Here's how the part is built. I have some questions about the finished solid (model axes, mm). A direction names the side the tool comes from. Give positions to 0.01 mm unless a question says otherwise; leave off trailing zeros. Write each loop counter-clockwise with the first axis right and the second up, starting at its lowest first coordinate (ties: lowest second). Pieces come first, ordered by that corner, then holes. Notation, with made-up numbers: (-36, -36.5) - (10, -36.5) arc R21 ccw to (10, -17.5) - close; hole circle Ø8 at (50.25, 22.25). An arc over 180 degrees is marked (long way). Write each question's results on one line, items separated by ' | '. Start each with the question number.
Item 1: Which directions (+Z, -Z, +X, -X, +Y, -Y) give clear straight access to the entire face, cutting with the end or side of a thin tool? Please do faces 1 (the flat face through (-102.855, 11, 2)), 2 (the flat face through (-101, -5.5, 2)), 3 (the flat face through (-24, -20.5, 3)).
Item 2: Suppose I cut it at C-C on x = -72.5. List the corners of the cut face in (y, z) for me, then the cut area to 3 significant figures.
Item 3: Suppose I cut it at A-A on z = 7.5. List the corners of the cut face in (x, y) for me.
Item 4: Will these pins go through, and if not, where does the flat tip stop? P1, Ø4, axis at x = -54.5, y = -14.5, coming from the +Z side; P2, Ø0.6, axis at x = -100.5, z = 10, coming from the +Y side; P3, Ø2.5, axis at x = 49, z = 8.5, coming from the -Y side.
Item 5: Suppose I cut it at B-B on y = -17.5. List the corners of the cut face in (x, z) for me.
Item 6: Please list where these lines run through material, in increasing order: line 1 along Y through (x, z) = (-8.5, 3); line 2 along X through (y, z) = (-16, 2.75); line 3 along X through (y, z) = (-8, 3.5).
Item 7: Suppose I cut it at D-D on y = 8. List the corners of the cut face in (x, z) for me.
Item 8: We'd pull the mould along Y, two halves only. Please class faces 4 (the flat face through (-102.855, -14, 2)), 5 (the flat face through (-26, -23.5, 2)), 6 (the flat face through (-26, -10.5, 3)): +Y half, -Y half, draft (parallel to the pull), parting line (faces both ways), or undercut.
```python
from build123d import *

# Parameters (mm, degrees)
F0_W     = 150
F0_H     = 3
F1_DEPTH = 5
F0_H_2   = 7
F2_DEPTH = 2
F3_DEPTH = 11
F5_W     = 2
F5_H     = 2
F6_DEPTH = 2
F7_R     = 1.5
F8_W     = 2
F8_H     = 2
F9_DEPTH = 2
F10_R    = 1.8


with BuildPart() as f1:
    # F0 (on Top) → F1 (new body)
    with BuildSketch(Plane.XY):
        Polygon((53.1447380781, 19.5), (-102.8552619219, 19.5), (-102.8552619219, 1.5), (-99.8552619219, 1.5), (-99.8552619219, 4.5), (-99.8552619219, 6.5), (-99.8552619219, 9.5), (-99.8552619219, 16.5), (50.1447380781, 16.5), (50.1447380781, 9.5), (50.1447380781, 6.5), (50.1447380781, 3), (50.1447380781, 0), (53.1447380781, 0), align=None)
        Polygon((-99.8552619219, 4.5), (-99.8552619219, 1.5), (-99.8552619219, -5.5), (-99.8552619219, -8.5), (-96.8552619219, -8.5), (-96.8552619219, 4.5), align=None)
        Polygon((-99.8552619219, -5.5), (-102.8552619219, -5.5), (-102.8552619219, -23.5), (53.1447380781, -23.5), (53.1447380781, -4), (50.1447380781, -4), (50.1447380781, -7), (50.1447380781, -10.5), (50.1447380781, -13.5), (50.1447380781, -20.5), (-99.8552619219, -20.5), (-99.8552619219, -13.5), (-99.8552619219, -10.5), (-99.8552619219, -8.5), align=None)
        with Locations((-24.8552619219, -12)):
            Rectangle(F0_W, F0_H)
        with Locations((-24.8552619219, 8)):
            Rectangle(F0_W, F0_H)
        Polygon((50.1447380781, -4), (50.1447380781, 0), (50.1447380781, 3), (47.1447380781, 3), (47.1447380781, -7), (50.1447380781, -7), align=None)
    extrude(amount=F1_DEPTH)

    # F0 (on Top) → F2 (join)
    with BuildSketch(Plane.XY):
        with Locations((-24.8552619219, 13)):
            Rectangle(F0_W, F0_H_2)
        Polygon((-99.8552619219, 6.5), (-99.8552619219, 4.5), (-96.8552619219, 4.5), (-96.8552619219, -8.5), (-99.8552619219, -8.5), (-99.8552619219, -10.5), (50.1447380781, -10.5), (50.1447380781, -7), (47.1447380781, -7), (47.1447380781, 3), (50.1447380781, 3), (50.1447380781, 6.5), align=None)
        with Locations((-24.8552619219, -17)):
            Rectangle(F0_W, F0_H_2)
    extrude(amount=F2_DEPTH)


with BuildPart() as f3:
    # F0 (on Top) → F3 (new body)
    with BuildSketch(Plane.XY):
        Polygon((-99.8552619219, 4.5), (-99.8552619219, 1.5), (-99.8552619219, -5.5), (-99.8552619219, -8.5), (-96.8552619219, -8.5), (-96.8552619219, 4.5), align=None)
    extrude(amount=F3_DEPTH)


with BuildPart() as f3b:
    # F0 (on Top) → F3, piece 2 (new body)
    with BuildSketch(Plane.XY):
        Polygon((50.1447380781, -4), (50.1447380781, 0), (50.1447380781, 3), (47.1447380781, 3), (47.1447380781, -7), (50.1447380781, -7), align=None)
    extrude(amount=F3_DEPTH)


with BuildPart() as f1_1:
    add(f1.part)

    # F4: union F3b, F3
    add(f3b.part)
    add(f3.part)

    # F5 (on face) → F6 (join)
    with BuildSketch(Plane(origin=(-99.8552619219, 0, 0), x_dir=(0, -1, 0), z_dir=(-1, 0, 0))):
        with Locations((2, 10)):
            Rectangle(F5_W, F5_H)
    extrude(amount=F6_DEPTH)

    # F7
    f7_edges = [f1_1.edges().sort_by_distance(p)[0] for p in [
        (-101.855262, -2, 11),
    ]]
    fillet(f7_edges, radius=F7_R)

    # F8 (on face) → F9 (join)
    with BuildSketch(Plane.YZ.offset(50.1447380781)):
        with Locations((-2, 10)):
            Rectangle(F8_W, F8_H)
    extrude(amount=F9_DEPTH)

    # F10
    f10_edges = [f1_1.edges().sort_by_distance(p)[0] for p in [
        (52.144738, -2, 11),
    ]]
    fillet(f10_edges, radius=F10_R)


solid = f1_1.part
```
Checked values:
1) face 1: +Z, -Z, -X, +Y, -Y | face 2: +Z, -Z, -X | face 3: +Z
2) outline: (-23.5, 0) - (19.5, 0) - (19.5, 5) - (16.5, 5) - (16.5, 2) - (9.5, 2) - (9.5, 5) - (6.5, 5) - (6.5, 2) - (-10.5, 2) - (-10.5, 5) - (-13.5, 5) - (-13.5, 2) - (-20.5, 2) - (-20.5, 5) - (-23.5, 5) - close | area: 122 mm^2
3) outline: (-99.86, -8.5) - (-96.86, -8.5) - (-96.86, 4.5) - (-99.86, 4.5) - close; (47.14, -7) - (50.14, -7) - (50.14, 3) - (47.14, 3) - close
4) P1: stops at z = 5 | P2: stops at y = -1 | P3: stops at y = -7
5) outline: (-102.86, 0) - (53.14, 0) - (53.14, 5) - (50.14, 5) - (50.14, 2) - (-99.86, 2) - (-99.86, 5) - (-102.86, 5) - close
6) line 1: y = -23.5 to -20.5, -13.5 to -10.5, 6.5 to 9.5, 16.5 to 19.5 | line 2: x = -102.86 to -99.86, 50.14 to 53.14 | line 3: x = -102.86 to -96.86, 50.14 to 53.14
7) outline: (-102.86, 0) - (53.14, 0) - (53.14, 5) - (-102.86, 5) - close
8) face 4: draft | face 5: -Y half | face 6: undercut
